from build123d import *

# Parameters (mm, degrees)
F0_W     = 38.1
F0_H     = 174.625
F1_DEPTH = 22.225
F3_DEPTH = 22.226
F4_DEPTH = 1.5875
F5_DEPTH = 1.5875


with BuildPart() as f1:
    # F0 (on Front) → F1 (new body)
    with BuildSketch(Plane.XZ):
        with Locations((19.05, 87.3125)):
            Rectangle(F0_W, F0_H)
    extrude(amount=F1_DEPTH)

    # F2 (on face) → F3 (cut, through all)
    with BuildSketch(Plane.XZ.offset(22.225)):
        Polygon((5.5413148632, 150.8125), (0, 173.0375), (0, 150.8125), align=None)
        Polygon((38.1, 150.8125), (38.1, 173.0375), (32.5586851368, 150.8125), align=None)
        Polygon((5.5413148632, 23.8125), (0, 23.8125), (0, 1.5875), align=None)
        Polygon((38.1, 1.5875), (38.1, 23.8125), (32.5586851368, 23.8125), align=None)
    extrude(amount=-F3_DEPTH, mode=Mode.SUBTRACT)

    # F4 (cut): a face of the model
    f4_faces = [f1.faces().sort_by_distance(p)[0] for p in [
        (19.05, -11.1125, 174.625),
    ]]
    extrude(f4_faces, amount=-F4_DEPTH, mode=Mode.SUBTRACT)

    # F5 (cut): a face of the model
    f5_faces = [f1.faces().sort_by_distance(p)[0] for p in [
        (19.05, -11.1125, 0),
    ]]
    extrude(f5_faces, amount=-F5_DEPTH, mode=Mode.SUBTRACT)


solid = f1.part
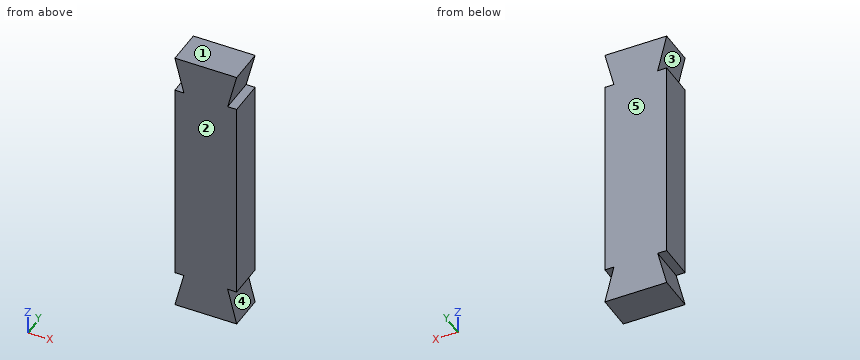
Model file for the job. Use its own axes, mm. Face numbers are marked on the shaded views. A direction names the side the tool comes from. Round coordinates to 2 decimals unless told otherwise and drop trailing zeros. Order: outer loops, then holes, each group sorted by start corner. A loop starts at its lowest first (then second) coordinate and runs counter-clockwise, first axis right, second up.
(1) Band-saw the part on D-D (z = 15). List the corners of the cut face in (x, y) (3 decimals), then the cut area to 3 significant figures.
(2) Pull direction Z, two halves, no side cores. Call the marked faces 1, 2 and 3: released by +Z, released by -Z, zero draft, split by the parting line, or undercut.
(3) Pin check, flat tip, straight feed: pin 1 (8 mm diameter, centred on y = -3, z = 89.5, fed in from -X). Stop position of the tip, or through.
(4) Band-saw the part on A-A (y = -7.25). List the corners of the cut face in (x, z), then the cut area to 3 significant figures.
(5) Band-saw the part on B-B (x = 3.5). List the corners of the cut face in (y, z) (1 decimal).
(6) 3-axis set-ups, long thin cutter, end or side, ignore diameter. For the marked faces 4 and 5: which of +Z, -Z, +X, -X, +Y, -Y reach the whole face in a straight line?
(7) Drill centre lines: line 1 (X direction, y = -18, z = 154.5); line 2 (X direction, y = -16.5, z = 11.5). Where is each one in solid material? Low to high.
(8) Band-saw the part on C-C (x = 35). List the corners of the cut face in (y, z) (1 decimal).
Verdict:
1. outline: (3.344, -22.225) - (34.756, -22.225) - (34.756, 0) - (3.344, 0) - close
1. area: 698 mm2
2. face 1: released by +Z
2. face 2: zero draft
2. face 3: undercut
3. pin 1: stops at x = 0
4. outline: (0, 1.59) - (38.1, 1.59) - (32.56, 23.81) - (38.1, 23.81) - (38.1, 150.81) - (32.56, 150.81) - (38.1, 173.04) - (0, 173.04) - (5.54, 150.81) - (0, 150.81) - (0, 23.81) - (5.54, 23.81) - close
4. area: 6,290 mm2
5. outline: (-22.2, 1.6) - (0, 1.6) - (0, 15.6) - (-22.2, 15.6) - close; (-22.2, 23.8) - (0, 23.8) - (0, 150.8) - (-22.2, 150.8) - close; (-22.2, 159) - (0, 159) - (0, 173) - (-22.2, 173) - close
6. face 4: +X, +Y, -Y
6. face 5: +Z, -Z, +X, -X, +Y
7. line 1: x = 4.62 to 33.48
7. line 2: x = 2.47 to 35.63
8. outline: (-22.2, 1.6) - (0, 1.6) - (0, 14) - (-22.2, 14) - close; (-22.2, 23.8) - (0, 23.8) - (0, 150.8) - (-22.2, 150.8) - close; (-22.2, 160.6) - (0, 160.6) - (0, 173) - (-22.2, 173) - close
